Part model, mm, in its own coordinate system. Give positions to 0.01 mm unless a question says otherwise; leave off trailing zeros. Order: outer loops, then holes, each group sorted by start corner. A loop starts at its lowest first (then second) coordinate and runs counter-clockwise, first axis right, second up. Notation, with made-up numbers: (46.5, 49.25) -> (103.5, 49.25) arc R16 cw to (103.5, 61.25) -> close; hole circle Ø3 at (27.25, 9.25). An arc over 180 degrees is marked (long way). Write item = value, one per line. Start each with the question number.
Item 1: Band-saw the part on A-A on z = 15.5. Write the cut outline in (x, y).
Item 2: Pull direction X, two halves, no side cores. Call faces 1 (the face through (22, 18, 20)), 2 (the face through (0, 22, 10)), 3 (the face through (21.183, 30.851, 14.304)), 4 (the face through (45, 22, 10)): +X half, -X half, draft (parallel to the pull), parting line (faces both ways), or undercut.
Item 3: Band-saw the part on B-B on z = 18.25. Write the cut outline in (x, y).
Item 4: Drill centre lines: line 1 along Y through (x, z) = (22.5, 8); line 2 along X through (y, z) = (14.5, 8.25); line 3 along X through (y, z) = (18.5, 11.5). Where is each one in solid material? Low to high.
```python
from build123d import *

# Parameters (mm, degrees)
F0_W     = 45
F0_H     = 45
F1_DEPTH = 20
F2_R     = 4.5763469256
F3_DEPTH = 25
F3_TAPER = -26.3


with BuildPart() as f1:
    # F0 (on Top) → F1 (new body)
    with BuildSketch(Plane.XY):
        with Locations((22.5, 22.5)):
            Rectangle(F0_W, F0_H)
    extrude(amount=F1_DEPTH)

    # F2 (on face) → F3 (cut)
    with BuildSketch(Plane.XY.offset(20)):
        with Locations((22.1453737468, 23.5223285854)):
            Circle(F2_R)
    extrude(amount=-F3_DEPTH, taper=F3_TAPER, mode=Mode.SUBTRACT)


solid = f1.part
```
Values found:
q1.outline = (0, 0) -> (45, 0) -> (45, 45) -> (0, 45) -> close; hole circle Ø13.6 at (22.15, 23.52)
q2.face_1 = draft
q2.face_2 = -X half
q2.face_3 = undercut
q2.face_4 = +X half
q3.outline = (0, 0) -> (45, 0) -> (45, 45) -> (0, 45) -> close; hole circle Ø10.88 at (22.15, 23.52)
q4.line_1 = 0 to 13.02, 34.02 to 45
q4.line_2 = 0 to 17.01, 27.29 to 45
q4.line_3 = 0 to 14.95, 29.34 to 45
